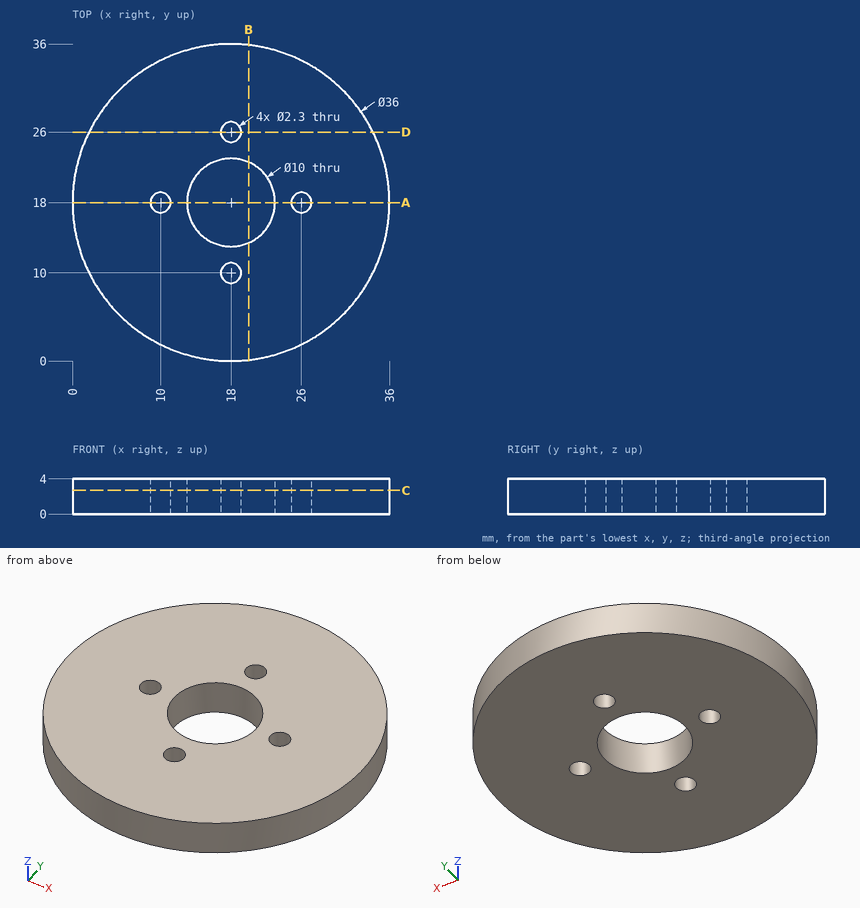
Drawing for the job (mm, zero at the part's lowest x, y, z). Round coordinates to 2 decimals unless told otherwise and drop trailing zeros. Write each loop counter-clockwise with the first axis right and the second up, starting at its lowest first coordinate (ties: lowest second). Pieces come first, ordered by that corner, then holes. Notation, with made-up numbers: M 39.25,-25 L 76.25,-25 A15 cw 76.25,-3 Z; hole C 63,27.25 d9. An arc over 180 degrees is marked long. Answer as a JSON object with one key per item and string values. Group by question number.
(1) Cut at D-D (y = 26). Give the cut face in (x, z), and give its area (3 significant figures).
(2) Cut at A-A (y = 18). Give the cut face in (x, z).
(3) Drill centre lines: L1, parallel to Y at x = 18, z = 1.7; L2, parallel to X at y = 20, z = 1.1; L3, parallel to Y at x = 26, z = 3.6. Where is each one in solid material? Low to high.
(4) Cut at C-C (z = 2.7). Give the cut face in (x, y).
(5) Flat gauge pins, fed straight in: pin 1 (1 mm diameter, centred on x = 26, z = 2, fed in from +Y); pin 2 (1.8 mm diameter, centred on x = 18, y = 26, fed in from +Z). Where does each tip first touch, or does it go through?
(6) Cut at B-B (x = 20). Give the cut face in (y, z).
Responses:
{
 "1": {"outline": "M 1.88,0 L 16.85,0 L 16.85,4 L 1.88,4 Z; M 19.15,0 L 34.12,0 L 34.12,4 L 19.15,4 Z", "area": "120 mm2"},
 "2": {"outline": "M 0,0 L 8.85,0 L 8.85,4 L 0,4 Z; M 11.15,0 L 13,0 L 13,4 L 11.15,4 Z; M 23,0 L 24.85,0 L 24.85,4 L 23,4 Z; M 27.15,0 L 36,0 L 36,4 L 27.15,4 Z"},
 "3": {"L1": "y = 0 to 8.85, 11.15 to 13, 23 to 24.85, 27.15 to 36", "L2": "x = 0.11 to 13.42, 22.58 to 35.89", "L3": "y = 1.88 to 16.85, 19.15 to 34.12"},
 "4": {"outline": "C 18,18 d36; hole C 10,18 d2.3; hole C 18,18 d10; hole C 18,10 d2.3; hole C 18,26 d2.3; hole C 26,18 d2.3"},
 "5": {"pin 1": "stops at y = 34.36", "pin 2": "passes through"},
 "6": {"outline": "M 0.11,0 L 13.42,0 L 13.42,4 L 0.11,4 Z; M 22.58,0 L 35.89,0 L 35.89,4 L 22.58,4 Z"}
}
